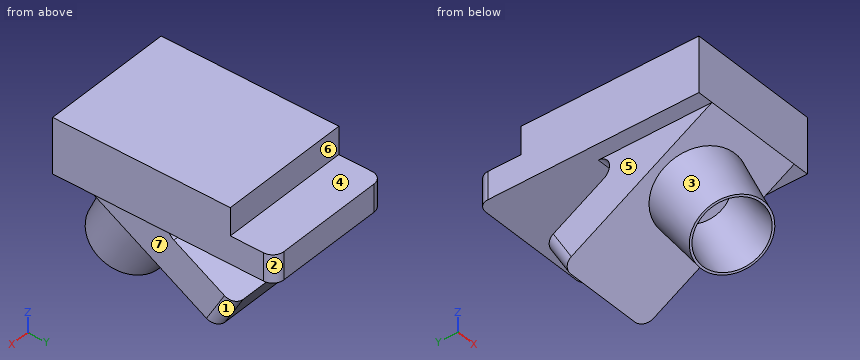
```python
from build123d import *

# Parameters (mm, degrees)
SKETCH1_W           = 23.75
SKETCH1_H           = 40
BOSS_EXTRUDE1_DEPTH = 10
SKETCH2_W           = 23.75
SKETCH2_H           = 8
CUT_EXTRUDE1_DEPTH  = 5
FILLET1_R           = 2
BOSS_EXTRUDE3_REACH = 44.573
SKETCH6_W           = 18
SKETCH6_H           = 6.5
SKETCH7_W           = 18
SKETCH7_H           = 6.5
CUT_EXTRUDE2_DEPTH  = 3.38
FILLET4_R           = 2
SKETCH8_R           = 7.5
BOSS_EXTRUDE4_DEPTH = 12
BOSS_EXTRUDE4_TAPER = 5
SKETCH9_R           = 5
CUT_EXTRUDE4_DEPTH  = 12
SKETCH10_R          = 5
CUT_EXTRUDE5_DEPTH  = 12
CUT_EXTRUDE5_DRAFT  = -5


with BuildPart() as part:
    # Sketch1 → Boss-Extrude1 (new body)
    with BuildSketch(Plane.XY):
        Rectangle(SKETCH1_W, SKETCH1_H)
    extrude(amount=-BOSS_EXTRUDE1_DEPTH)

    # Sketch2 → Cut-Extrude1 (cut)
    with BuildSketch(Plane.XY):
        with Locations((0, 16)):
            Rectangle(SKETCH2_W, SKETCH2_H)
    extrude(amount=-CUT_EXTRUDE1_DEPTH, mode=Mode.SUBTRACT)

    # Fillet1
    fillet1_edges = [part.edges().sort_by_distance(p)[0] for p in [
        (-11.875, 20, -7.5),
        (11.875, 20, -7.5),
    ]]
    fillet(fillet1_edges, radius=FILLET1_R)

    # Boss-Extrude3: up to this plane
    boss_extrude3_end = Plane(origin=(0, 0, -10), z_dir=(0, 0, -1))
    # Sketch6 → Boss-Extrude3 (add, up to the surface)
    with BuildSketch(Plane(origin=(0, 19.330127019, -11.160254038), x_dir=(-1, 0, 0), z_dir=(0, -0.866025403784438, 0.500000000000001)), mode=Mode.PRIVATE) as boss_extrude3_sk1:
        with Locations((0, 15.410254038)):
            Rectangle(SKETCH6_W, SKETCH6_H)
    boss_extrude3_tool1 = split(extrude(boss_extrude3_sk1.sketch, amount=BOSS_EXTRUDE3_REACH, mode=Mode.PRIVATE), bisect_by=boss_extrude3_end, keep=Keep.BOTH, mode=Mode.PRIVATE)
    add(boss_extrude3_tool1.solids().sort_by_distance((0, 11.625, -24.505926))[0])

    # Sketch7 → Cut-Extrude2 (cut)
    with BuildSketch(Plane(origin=(0, 19.330127019, -11.160254038), x_dir=(1, 0, 0), z_dir=(0, 0.866025403784438, -0.5000000000000012))):
        with Locations((0, 15.410254038)):
            Rectangle(SKETCH7_W, SKETCH7_H)
    extrude(amount=-CUT_EXTRUDE2_DEPTH, mode=Mode.SUBTRACT)

    # Fillet4
    fillet4_edges = [part.edges().sort_by_distance(p)[0] for p in [
        (0, -7, -10),
        (9, 8.697834135, -22.815925513),
        (-9, 8.697834135, -22.815925513),
    ]]
    fillet(fillet4_edges, radius=FILLET4_R)

    # Sketch8 → Boss-Extrude4 (add)
    with BuildSketch(Plane(origin=(0, -9.330127019, -16.160254038), x_dir=(-1, 0, 0), z_dir=(0, -0.500000000000001, -0.8660254037844382))):
        with Locations((0, -1.020508076)):
            Circle(SKETCH8_R)
    extrude(amount=BOSS_EXTRUDE4_DEPTH, taper=BOSS_EXTRUDE4_TAPER)

    # Sketch9 → Cut-Extrude4 (cut)
    with BuildSketch(Plane(origin=(0, -15.330127019, -26.552558883), x_dir=(-1, 0, 0), z_dir=(0, -0.5000000000000011, -0.8660254037844382))):
        with Locations(Location((0, -1.020508076, 0), (0, 0, 90))):
            Circle(SKETCH9_R)
    extrude(amount=-CUT_EXTRUDE4_DEPTH, mode=Mode.SUBTRACT)


with BuildPart() as cut_extrude5_tool:
    # Sketch10 → Cut-Extrude5 (with draft: the straight prism first)
    with BuildSketch(Plane(origin=(0, -9.330127019, -16.160254038), x_dir=(-1, 0, 0), z_dir=(0, -0.5000000000000012, -0.866025403784438))):
        with Locations((0, -1.020508076)):
            Circle(SKETCH10_R)
    extrude(amount=CUT_EXTRUDE5_DEPTH)
    # Cut-Extrude5: the draft: its side faces are tilted about the plane it starts from
    cut_extrude5_sides = [cut_extrude5_tool.faces().sort_by_distance(p)[0] for p in [
        (5, -13.213912937, -20.846152423),
    ]]
    draft(cut_extrude5_sides, Plane(origin=(0, -9.330127019, -16.160254038), x_dir=(-1, 0, 0), z_dir=(0, -0.5000000000000012, -0.866025403784438)), CUT_EXTRUDE5_DRAFT)


with BuildPart() as part_1:
    add(part.part)

    # Cut-Extrude5: cut by cut_extrude5_tool
    add(cut_extrude5_tool.part, mode=Mode.SUBTRACT)


solid = part_1.part
```
Check sheet for the modelled part. Datum: model origin and axes. Units: mm. Face numbers are marked on the shaded views. A direction names the side the tool comes from. Coordinates: 2 decimals unless noted, no trailing zeros. Order: outer loops, then holes, each group sorted by start corner. A loop starts at its lowest first (then second) coordinate and runs counter-clockwise, first axis right, second up. Notation, with made-up numbers: M 64,7 L 79,7 A34 cw 79,46 Z; hole C 57,-3 d11. An arc over 180 degrees is marked long. Write each question's results on one line, items separated by ' | '. Start each with the question number.
1. Cross-section at A-A on y = 0. Record the cut outline in (x, z) (3 decimals).
2. Cross-section at B-B on z = -21. State how many separate pieces and enclosed holes the cut face has, and give its area (3 significant figures).
3. Mould release check, pull along Z, two halves, no side actions. Record for the marked faces 1, 2, 3 and 4: +Z half, -Z half, draft (parallel to the pull), parting line (faces both ways), or undercut.
4. Go/stop test with flat-tipped pins: P1, Ø6.5, axis at x = -3.5, y = 17, coming from the +Z side; P2, Ø3, axis at y = 5.5, z = -18, coming from the +X side; P3, Ø2.5, axis at x = 0, z = -3.5, coming from the +Y side; P4, Ø1.5, axis at x = 6.5, y = -12.5, coming from the +Z side. Record where each tip stops, or that it passes through.
5. Material ranges on probe 1 along Y at (x, z) = (-1.75, -19.5); probe 2 along Y at (x, z) = (-2.5, -20.5); probe 3 along X at (y, z) = (-9, -19.5), recorded low to high.
6. Cross-section at C-C on x = 8.25. Record the cut outline in (y, z), and give its area (3 significant figures).
7. Cross-section at D-D on z = -2.75. Record the cut outline in (x, y) (3 decimals), and give its area (3 significant figures).
8. Access from +Z, -Z, +X, -X, +Y, -Y to the whole of each face (thin tool, end or side, straight path). Record for the marked faces 5, 6 and 7.
Checks:
1) outline: M -11.875,-10 L -9,-10 L -9,-10.055 L 9,-10.055 L 9,-10 L 11.875,-10 L 11.875,0 L -11.875,0 Z; M -9,-21.547 L 9,-21.547 L 9,-14.041 L -9,-14.041 Z
2) separate pieces: 2 | enclosed holes: 1 | area: 255 mm²
3) face 1: -Z half | face 2: draft | face 3: undercut | face 4: +Z half
4) P1: stops at z = -5 | P2: stops at x = 9 | P3: stops at y = 12 | P4: stops at z = 0
5) probe 1: y = -20 to -18.65, -6.85 to -4.04, -3.55 to 9.45 | probe 2: y = -20.19 to -19, -7.67 to -5.02, -1.81 to 10.03 | probe 3: x = -6.62 to -4.31, 4.31 to 6.62
6) outline: M -20,-10 L 6.69,-25.41 L 9.94,-19.78 L -0.54,-13.73 A2 cw 0.46,-10 L 20,-10 L 20,-5 L 12,-5 L 12,0 L -20,0 Z | area: 533 mm²
7) outline: M -11.875,-20 L 11.875,-20 L 11.875,12 L -11.875,12 Z | area: 760 mm²
8) face 5: -Z, -X, +Y, -Y | face 6: +Z, +X, -X, +Y | face 7: -Z, +X, +Y, -Y
